Input: part model. Units: mm. Frame: model coordinates. Coordinates: 2 decimals unless noted, no trailing zeros. Write each loop counter-clockwise with the first axis right and the second up, starting at its lowest first coordinate (ties: lowest second). Pieces come first, ordered by that corner, then holes. Notation, with made-up numbers: (14.5, 13.5) -> (68.5, 13.5) arc R3 ccw to (68.5, 17.5) -> close; hole circle Ø9 at (-6.75, 77). An arc over 180 degrees is marked (long way). Use one line per item in the form item = value. Start each with the question number.
(1) Ray query, line 1 along Z through (x, y) = (9.05, 0); line 2 along X through (y, z) = (-0.5, -75); line 3 along Z through (x, y) = (-8.75, -0.75). Return the intervals inside material, ascending.
(2) First-contact query: pin 1 (1.5 mm diameter, centred on y = -1, z = 0, fed in from -X); pin 2 (1.5 mm diameter, centred on y = -3, z = -40.5, fed in from -X); pin 3 (1.5 mm diameter, centred on y = -2.5, z = -34, fed in from -X). Flat tips, straight axial feed; report the tip coordinate or a pass-through.
(3) Cut plane A-A on y = 0. Return the cut outline in (x, z), plus the area to 4 significant figures.
(4) Cut plane C-C on z = 87.75. Return the cut outline in (x, y), plus the area to 3 significant figures.
(5) Cut plane D-D on z = 7.5. Return the cut outline in (x, y), plus the area to 3 significant figures.
(6) Cut plane B-B on x = 0. Return the cut outline in (y, z).
```python
from build123d import *

# Parameters (mm, degrees)
SKETCH1_R           = 10
SKETCH1_R_2         = 8.5
BOSS_EXTRUDE1_DEPTH = 100.25
SKETCH2_R           = 2
CUT_EXTRUDE1_DEPTH  = 102.242592322


with BuildPart() as part:
    # Sketch1 → Boss-Extrude1 (new body)
    with BuildSketch(Plane.XY):
        with Locations(Location((0, 0, 0), (0, 0, 180))):
            Circle(SKETCH1_R)
        with Locations(Location((0, 0, 0), (0, 0, 180))):
            Circle(SKETCH1_R_2, mode=Mode.SUBTRACT)
    boss_extrude1 = extrude(amount=BOSS_EXTRUDE1_DEPTH)

    # Sketch2 → Cut-Extrude1 (cut, symmetric)
    with BuildSketch(Plane(origin=(0, 0, 0), x_dir=(0, 0, -1), z_dir=(1, 0, 0))):
        with Locations((-87.75, 0)):
            Circle(SKETCH2_R)
    cut_extrude1 = extrude(amount=CUT_EXTRUDE1_DEPTH, both=True, mode=Mode.SUBTRACT)

    # Mirror1: Boss-Extrude1, Cut-Extrude1 across plane
    add(boss_extrude1.mirror(Plane.XY))
    add(cut_extrude1.mirror(Plane.XY), mode=Mode.SUBTRACT)


solid = part.part
```
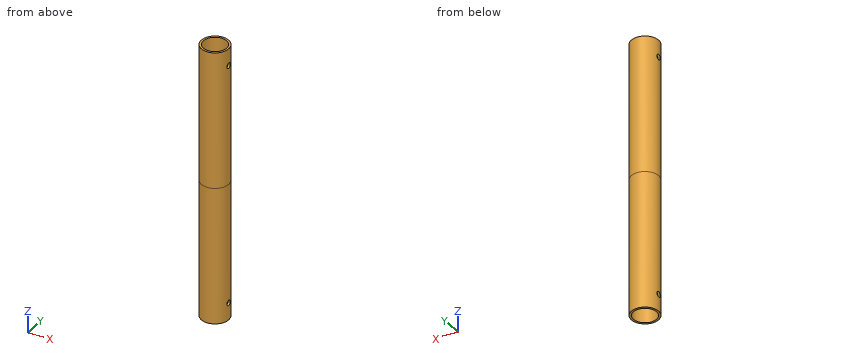
Values:
q1.line_1 = -100.25 to -89.75, -85.75 to 85.75, 89.75 to 100.25
q1.line_2 = -9.99 to -8.49, 8.49 to 9.99
q1.line_3 = -100.25 to -89.6, -85.9 to 85.9, 89.6 to 100.25
q2.pin_1 = -10
q2.pin_2 = -9.74
q2.pin_3 = -9.85
q3.outline = (-10, -100.25) -> (-8.5, -100.25) -> (-8.5, -89.75) -> (-10, -89.75) -> close; (-10, -85.75) -> (-8.5, -85.75) -> (-8.5, 85.75) -> (-10, 85.75) -> close; (-10, 89.75) -> (-8.5, 89.75) -> (-8.5, 100.25) -> (-10, 100.25) -> close; (8.5, -100.25) -> (10, -100.25) -> (10, -89.75) -> (8.5, -89.75) -> close; (8.5, -85.75) -> (10, -85.75) -> (10, 85.75) -> (8.5, 85.75) -> close; (8.5, 89.75) -> (10, 89.75) -> (10, 100.25) -> (8.5, 100.25) -> close
q3.area = 577.5 mm2
q4.outline = (-9.8, -2) arc R10 ccw to (9.8, -2) -> (8.26, -2) arc R8.5 cw to (-8.26, -2) -> close; (-9.8, 2) -> (-8.26, 2) arc R8.5 cw to (8.26, 2) -> (9.8, 2) arc R10 ccw to start
q4.area = 75.1 mm2
q5.outline = circle Ø20 at (0, 0); hole circle Ø17 at (0, 0)
q5.area = 87.2 mm2
q6.outline = (-10, -100.25) -> (-8.5, -100.25) -> (-8.5, 100.25) -> (-10, 100.25) -> close; (8.5, -100.25) -> (10, -100.25) -> (10, 100.25) -> (8.5, 100.25) -> close
